from build123d import *

# Parameters (mm, degrees)
SKETCH1_R           = 12
BOSS_EXTRUDE1_DEPTH = 2.5
CUT_EXTRUDE2_DEPTH  = 18.691806013
CIRPATTERN2_COUNT   = 10
SKETCH3_R           = 2
CUT_EXTRUDE3_DEPTH  = 18.349304428
BOSS_EXTRUDE2_START = 0.5
SKETCH4_R           = 6.5
SKETCH4_R_2         = 6
SKETCH4_R_3         = 3.5
SKETCH4_R_4         = 2
BOSS_EXTRUDE2_DEPTH = 0.5


with BuildPart() as part:
    # Sketch1 → Boss-Extrude1 (new, symmetric)
    with BuildSketch(Plane.XY):
        Circle(SKETCH1_R)
    extrude(amount=BOSS_EXTRUDE1_DEPTH, both=True)

    # Sketch2 → Cut-Extrude2 (cut, through all)
    with BuildSketch(Plane.XY.offset(2.5)):
        with BuildLine():
            ThreePointArc((1.173656282, 7.407599539), (0, 7.5), (-1.173656282, 7.407599539))
            ThreePointArc((-1.173656282, 7.407599539), (-1.669021324, 9.83476625), (-3.49865822, 11.504782295))
            ThreePointArc((-3.49865822, 11.504782295), (0, 12.025), (3.49865822, 11.504782295))
            ThreePointArc((3.49865822, 11.504782295), (1.669021324, 9.83476625), (1.173656282, 7.407599539))
        make_face()
    cut_extrude2 = extrude(amount=-CUT_EXTRUDE2_DEPTH, mode=Mode.SUBTRACT)

    # CirPattern2: Cut-Extrude2 ×10 about axis
    cirpattern2_axis = Axis((0, 0, 0), (0, 0, 1))
    for i in range(1, CIRPATTERN2_COUNT):
        add(cut_extrude2.rotate(cirpattern2_axis, i * 360 / CIRPATTERN2_COUNT), mode=Mode.SUBTRACT)

    # Sketch3 → Cut-Extrude3 (cut, through all)
    with BuildSketch(Plane.XY.offset(2.5)):
        Circle(SKETCH3_R)
    extrude(amount=-CUT_EXTRUDE3_DEPTH, mode=Mode.SUBTRACT)

    # Sketch4 → Boss-Extrude2 (add)
    # profile 1 of 2: a face of its own
    with BuildSketch(Plane.XY.offset(2.5).offset(BOSS_EXTRUDE2_START)):
        Circle(SKETCH4_R)
        Circle(SKETCH4_R_2, mode=Mode.SUBTRACT)
    # profile 2 of 2: a face of its own
    with BuildSketch(Plane.XY.offset(2.5).offset(BOSS_EXTRUDE2_START)):
        Circle(SKETCH4_R_3)
        Circle(SKETCH4_R_4, mode=Mode.SUBTRACT)
    boss_extrude2 = extrude(amount=-BOSS_EXTRUDE2_DEPTH)

    # Mirror1: Boss-Extrude2 across plane
    add(boss_extrude2.mirror(Plane.XY))


solid = part.part
Model file for the job. Use its own axes, mm. A direction names the side the tool comes from. Coordinates: 2 decimals unless noted, no trailing zeros. Write each loop counter-clockwise with the first axis right and the second up, starting at its lowest first coordinate (ties: lowest second). Pieces come first, ordered by that corner, then holes. Notation, with made-up numbers: (18.25, 45) -> (76.25, 45) arc R28 ccw to (76.25, 63) -> close; hole circle Ø3 at (42, -28). An arc over 180 degrees is marked (long way). One line per item, written item: value. Start each with the question number.
1) Slice it at B-B on y = 9.75. Write the cut outline in (x, z).
2) Probe probe 1 along Y at (x, z) = (0, -2.6); probe 2 along Y at (x, z) = (0, 0.55); probe 3 along X at (y, z) = (6, 0.15). List the from-to ranges inside material, lowest first.
3) Pull direction Y, two halves, no side cores. Call faces 1 (the face through (2, -2, 3)), 2 (the face through (-5.158, -3.955, -2.754)), 3 (the face through (3.233, -1.341, -2.754)): +Y half, -Y half, draft (parallel to the pull), parting line (faces both ways), or undercut.
4) Slice it at C-C on x = -7. Write the cut outline in (y, z), then the cut area to 3 significant figures.
5) Slice it at D-D on x = 2.5. Write the cut outline in (y, z), then the cut area to 3 significant figures.
6) Flat gauge pins, fed straight in: pin 1 Ø3 at (y, z) = (-6, -2) entering from +X; pin 2 Ø13 at (x, y) = (1, 1.5) entering from -Z; pin 3 Ø1 at (y, z) = (-6, 1) entering from +X; pin 4 Ø2 at (x, y) = (6, -5) entering from +Z. Where does each tip first touch, or does it go through?
7) Which spindle directions (+Z, -Z, +X, -X, +Y, -Y) get a long thin tool onto all of the face, cutting with end or side? Do faces 4 (the face through (0, -2, 0)), 5 (the face through (3.233, -1.341, 2.754)), 6 (the face through (3, -3, -2.5)). Say none if no direction does.
Answers follow:
1. outline: (-4.44, -2.5) -> (-1.62, -2.5) -> (-1.62, 2.5) -> (-4.44, 2.5) -> close; (1.62, -2.5) -> (4.44, -2.5) -> (4.44, 2.5) -> (1.62, 2.5) -> close
2. probe 1: -6.5 to -6, -3.5 to -2, 2 to 3.5, 6 to 6.5
2. probe 2: -7.5 to -2, 2 to 7.5
2. probe 3: -9.66 to -5.8, -4.5 to 4.5, 5.8 to 9.66
3. face 1: draft
3. face 2: parting line
3. face 3: undercut
4. outline: (-6.91, -2.5) -> (-3.48, -2.5) -> (-3.48, 2.5) -> (-6.91, 2.5) -> close; (-2.69, -2.5) -> (2.69, -2.5) -> (2.69, 2.5) -> (-2.69, 2.5) -> close; (3.48, -2.5) -> (6.91, -2.5) -> (6.91, 2.5) -> (3.48, 2.5) -> close
4. area: 61.2 mm2
5. outline: (-10.86, -2.5) -> (-6, -2.5) -> (-6, -3) -> (-5.45, -3) -> (-5.45, -2.5) -> (-2.45, -2.5) -> (-2.45, -3) -> (2.45, -3) -> (2.45, -2.5) -> (5.45, -2.5) -> (5.45, -3) -> (6, -3) -> (6, -2.5) -> (10.86, -2.5) -> (10.86, 2.5) -> (6, 2.5) -> (6, 3) -> (5.45, 3) -> (5.45, 2.5) -> (2.45, 2.5) -> (2.45, 3) -> (-2.45, 3) -> (-2.45, 2.5) -> (-5.45, 2.5) -> (-5.45, 3) -> (-6, 3) -> (-6, 2.5) -> (-10.86, 2.5) -> close
5. area: 115 mm2
6. pin 1: x = 9.86
6. pin 2: z = -3
6. pin 3: x = 9.8
6. pin 4: z = 2.5
7. face 4: +Z, -Z
7. face 5: +Z
7. face 6: -Z
